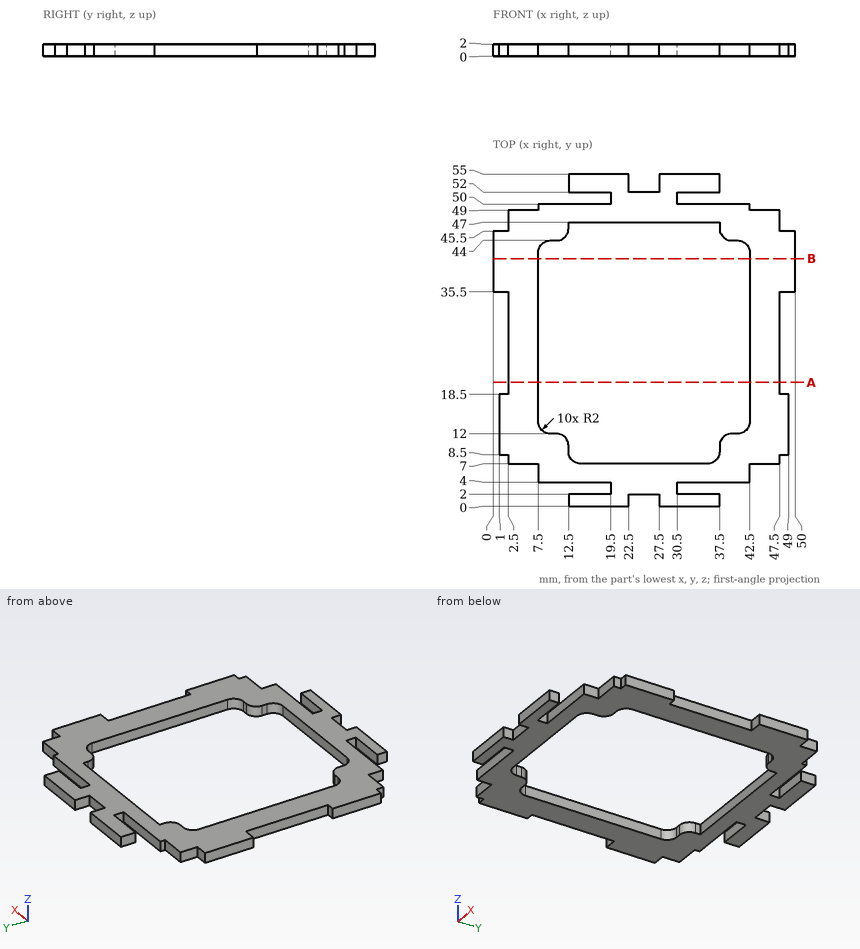
The drawing under review shows one solid part. Ordinate dimensions are in mm from its lowest x, y, z. Coordinates: 2 decimals unless noted, no trailing zeros. Loops run counter-clockwise (first coordinate to the right, second up) from the corner with the lowest first, then second, coordinate; pieces in that order, holes last. Notation, with made-up numbers: (8, -3) - (43, -3) arc R33 cw to (43, 33) - close; hole circle Ø11 at (57, 82). An arc over 180 degrees is marked (long way). Use CSV: the item, a comma, the result in double quotes. Start each with the question number.
1. Add section B-B on y = 41. Give the boundary of the cut face in (x, z), plus the area to 3 significant figures.
2. Add section A-A on y = 20.5. Give the boundary of the cut face in (x, z), plus the area to 3 significant figures.
3. To check wall thickness, follow probe 1 along Y at (x, z) = (32.5, 0.7); probe 2 along Y at (x, z) = (29, 0.85); probe 3 along Y at (x, z) = (10, 1.9). State the ranges of each line that lie inside material, in increasing order.
4. Clearance check with flat-ended pins moving along their axes: pin 1 (1 mm diameter, centred on y = 7, z = 0.5, fed in from +X); pin 2 (1 mm diameter, centred on x = 4, z = 1, fed in from +Y); pin 3 (0.6 mm diameter, centred on y = 0.5, z = 0.5, fed in from +X). State where each tip first meets the part, or that it passes through.
Resolved:
1,outline,"(0, 0) - (7.5, 0) - (7.5, 2) - (0, 2) - close; (42.5, 0) - (50, 0) - (50, 2) - (42.5, 2) - close"
1,area,"30.0 mm2"
2,outline,"(2.5, 0) - (7.5, 0) - (7.5, 2) - (2.5, 2) - close; (42.5, 0) - (47.5, 0) - (47.5, 2) - (42.5, 2) - close"
2,area,"20.0 mm2"
3,probe 1,"0 to 2, 4 to 7, 47 to 50, 52 to 55"
3,probe 2,"0 to 7, 47 to 55"
3,probe 3,"4 to 12, 44 to 50"
4,pin 1,"x = 47.5"
4,pin 2,"y = 49"
4,pin 3,"x = 37.5"
